from build123d import *

# Parameters (mm, degrees)
SKETCH1_W                = 0.3
SKETCH1_H                = 0.3
BOSS_EXTRUDE1_DEPTH      = 4
SKETCH1_5_W              = 0.3
SKETCH1_5_H              = 0.3
BOSS_EXTRUDE2_DEPTH      = 4
BOSS_EXTRUDE3_DEPTH      = 3
BOSS_EXTRUDE4_DEPTH      = 3.00199999
BOSS_EXTRUDE4_DEPTH_BACK = 0.99800001
SKETCH3_W                = 4.5
SKETCH3_H                = 3.5
CUT_EXTRUDE1_DEPTH       = 4


with BuildPart() as part:
    # Sketch1 → Boss-Extrude1 (new body)
    with BuildSketch(Plane(origin=(0, 0, 0), x_dir=(1, 0, 0), z_dir=(0, 1, 0))):
        Polygon((2.114911513, 12.894399988), (-14.885088487, 12.894399988), (-16.417177373, 11.608824769), (-10.632088886, 4.714424781), (0, -3), (47.2, -2), (48.485575219, -1.532088886), (57.239858961, 5.813627372), (55.954283741, 7.345716259), (50.8, 12.5), (24.8, 12.5), (24.8, 3.5), (14.8, 3.5), (14.8, 0), (2.114911513, 0), align=None)
        Polygon((47.392836283, -0.229813333), (47.30919107, -0.3), (47.2, -0.3), (47.2, 0), align=None, mode=Mode.SUBTRACT)
        with Locations((-0.15, -0.15)):
            Rectangle(SKETCH1_W, SKETCH1_H, mode=Mode.SUBTRACT)
    extrude(amount=BOSS_EXTRUDE1_DEPTH)

    # Sketch1_5 → Boss-Extrude2 (add)
    with BuildSketch(Plane(origin=(0, 0, 0), x_dir=(1, 0, 0), z_dir=(0, 1, 0))):
        with Locations((-0.15, -0.15)):
            Rectangle(SKETCH1_5_W, SKETCH1_5_H)
        Polygon((47.2, 0), (47.2, -0.3), (47.30919107, -0.3), (47.392836283, -0.229813333), align=None)
    extrude(amount=BOSS_EXTRUDE2_DEPTH)

    # Sketch1_6 → Boss-Extrude3 (add)
    with BuildSketch(Plane(origin=(0, 0, 0), x_dir=(1, 0, 0), z_dir=(0, 1, 0))):
        with BuildLine():
            Line((-0.3, -0.3), (-0.3, 4.117528082))
            ThreePointArc((-0.3, 4.117528082), (-0.885786438, 5.114213562), (-1.882471918, 5.7))
            Line((-1.882471918, 5.7), (-9.239892297, 5.7))
            Line((-9.239892297, 5.7), (-15.11490182, 12.701563705))
            Line((-15.11490182, 12.701563705), (-16.417177373, 11.608824769))
            Line((-16.417177373, 11.608824769), (-10.632088886, 4.714424781))
            Line((-10.632088886, 4.714424781), (0, -3))
            Line((0, -3), (47.2, -2))
            Line((47.2, -2), (48.485575219, -1.532088886))
            Line((48.485575219, -1.532088886), (57.239858961, 5.813627372))
            Line((57.239858961, 5.813627372), (56.147120024, 7.115902926))
            Line((56.147120024, 7.115902926), (47.30919107, -0.3))
            Line((47.30919107, -0.3), (38.858723672, -0.3))
            Line((38.858723672, -0.3), (38.858723672, 0.607136774))
            ThreePointArc((38.858723672, 0.607136774), (33.95, 4.199275448), (29.041276328, 0.607136774))
            Line((29.041276328, 0.607136774), (29.041276328, -0.3))
            Line((29.041276328, -0.3), (-0.3, -0.3))
        make_face()
    extrude(amount=-BOSS_EXTRUDE3_DEPTH)

    # Sketch2 → Boss-Extrude4 (add, two sides: drawn at the far end of the back side and taken through both)
    with BuildSketch(Plane(origin=(0, -3, 0), x_dir=(-1, 0, 0), z_dir=(0, -1, 0)).offset(-BOSS_EXTRUDE4_DEPTH_BACK)):
        Polygon((-55.954283741, 7.345716259), (-57.239858961, 5.813627372), (-48.485575219, -1.532088886), (-47.2, -2), (0, -3), (10.632088886, 4.714424781), (16.417177373, 11.608824769), (14.885088487, 12.894399988), (13.295498156, 11), (-6, 11), (-6, 5.000587023), (-21.8, 5.000587023), (-21.8, 11), (-51.796266659, 11), (-51.796266659, 3.856725658), align=None)
    extrude(amount=BOSS_EXTRUDE4_DEPTH + BOSS_EXTRUDE4_DEPTH_BACK)

    # Sketch3 → Cut-Extrude1 (cut)
    with BuildSketch(Plane(origin=(0, 4, 0), x_dir=(1, 0, 0), z_dir=(0, 1, 0))):
        with Locations((17.05, 1.75)):
            Rectangle(SKETCH3_W, SKETCH3_H)
    extrude(amount=-CUT_EXTRUDE1_DEPTH, mode=Mode.SUBTRACT)


solid = part.part
Read the model definition and answer for the solid it produces. Units are mm, in the model's axes. A direction names the side the tool comes from. Give positions to 0.01 mm unless a question says otherwise; leave off trailing zeros. Write each loop counter-clockwise with the first axis right and the second up, starting at its lowest first coordinate (ties: lowest second). Pieces come first, ordered by that corner, then holes. Notation, with made-up numbers: (-11.75, 54) -> (-2.75, 54) arc R14 ccw to (-2.75, 79) -> close; hole circle Ø10 at (49.25, 80.5). An arc over 180 degrees is marked (long way). Answer as a JSON object with one key per item and string values. Group by question number.
1) Find section C-C (z = -8.75). Write down the section's boundary in (x, y), and give its area (3 significant figures).
2) Consider L1, parallel to Y at x = 26.5, z = -5; L2, parallel to X at y = -3, z = -5.75; L3, parallel to Y at x = 19, z = -3.75. Determine where each line is inside the solid, lowest interval first. Write a range as from..to.
3) Each of these flat-tipped pins is pushed along its axis until it touches: P1, Ø1, axis at x = -4.5, y = -1, coming from the -Z side; P2, Ø1.2, axis at x = 9.5, y = 3, coming from the -Z side; P3, Ø0.7, axis at y = -1.5, z = -0.5, coming from the -X side. Where does it stop, or does it pass through?
4) A tool of negligible diameter and unlimited length cuts with its end or side. For faces 4 (the flat face through (38, 2, -12.5)), 5 (the flat face through (-6, -1, -5.7)), 6 (the flat face through (6, -4, -8)), 7 (the flat face through (11, 2, 0)), from which of +Z, -Z, +X, -X, +Y, -Y can it reach the whole face along a straight path? Write none if from no direction.
5) Find section B-B (y = -5). Write down the section's boundary in (x, z), and give its area (3 significant figures).
6) Find section A-A (z = -2.25). Write down the section's boundary in (x, y).
7) The mould has two halves that part along X. Classify faces 1 (the flat face through (-4, -4, -11)), 2 (the flat face through (-13.48, -0.93, -8.11)), 3 (the flat face through (21, -2.002, -3)): +X half, -X half, draft (parallel to the pull), parting line (faces both ways), or undercut.
8) Find section D-D (x = 30). Write down the section's boundary in (y, z), and give its area (3 significant figures).
Values follow:
{
 "1": {"outline": "(-14.02, -6) -> (6, -6) -> (6, -2) -> (-11.8, -2) -> (-11.8, 0) -> (2.11, 0) -> (2.11, 4) -> (-14.02, 4) -> close; (21.8, -6) -> (51.8, -6) -> (51.8, -2) -> (21.8, -2) -> close; (24.8, 0) -> (54.55, 0) -> (54.55, 4) -> (24.8, 4) -> close", "area": "388 mm2"},
 "2": {"L1": "y = -6..-2, 0..4", "L2": "x = -11.5..6, 21.8..51.8, 54.05..57.16", "L3": "y = -6..-2"},
 "3": {"P1": "stops at z = -5.7", "P2": "stops at z = 0", "P3": "stops at x = -5.31"},
 "4": {"face 4": "-Z, +X, +Y, -Y", "face 5": "-Z", "face 6": "-Z, +Y, -Y", "face 7": "-Z, +Y"},
 "5": {"outline": "(-16.42, -11.61) -> (-14.89, -12.89) -> (-13.3, -11) -> (6, -11) -> (6, -5) -> (21.8, -5) -> (21.8, -11) -> (51.8, -11) -> (51.8, -3.86) -> (55.95, -7.35) -> (57.24, -5.81) -> (48.49, 1.53) -> (47.2, 2) -> (0, 3) -> (-10.63, -4.71) -> close", "area": "736 mm2"},
 "6": {"outline": "(-7.24, -6) -> (52.99, -6) -> (52.99, 4) -> (19.3, 4) -> (19.3, 0) -> (29.92, 0) -> (29.92, -2) -> (-0.3, -2) -> (-0.3, 0) -> (2.11, 0) -> (2.11, 4) -> (-7.24, 4) -> close; hole (37.98, -2) -> (50.35, -2) -> (50.35, 0) -> (37.98, 0) -> close"},
 "7": {"face 1": "draft", "face 2": "-X half", "face 3": "undercut"},
 "8": {"outline": "(-6, -11) -> (-2, -11) -> (-2, -2.35) -> (0, -2.35) -> (0, -12.5) -> (4, -12.5) -> (4, 2.36) -> (-6, 2.36) -> close", "area": "122 mm2"}
}
